```python
from build123d import *

# Parameters (mm, degrees)
SKETCH1_W                    = 40
SKETCH1_H                    = 60
SKETCH1_R                    = 2
BASE_FLANGE1_DEPTH           = 2
EDGE_FLANGE1_STRIP_W         = 9.4732
EDGE_FLANGE1_STRIP_H         = 2
EDGE_FLANGE1_STRIP_CUT_DEPTH = 40
EDGE_FLANGE1_DEPTH           = 40
SKETCH7_R                    = 2
CUT_EXTRUDE1_DEPTH           = 10


# Sheet-metal steps are written as plain solids
with BuildPart() as part:
    # Sketch1 → Base-Flange1 (new body)
    with BuildSketch(Plane.XY):
        with Locations((0, 30)):
            Rectangle(SKETCH1_W, SKETCH1_H)
        with Locations((-14, 50)):
            Circle(SKETCH1_R, mode=Mode.SUBTRACT)
        with Locations((0, 50)):
            Circle(SKETCH1_R, mode=Mode.SUBTRACT)
        with Locations((14, 50)):
            Circle(SKETCH1_R, mode=Mode.SUBTRACT)
        with Locations((-7, 40)):
            Circle(SKETCH1_R, mode=Mode.SUBTRACT)
        with Locations((7, 40)):
            Circle(SKETCH1_R, mode=Mode.SUBTRACT)
        with Locations((-14, 30)):
            Circle(SKETCH1_R, mode=Mode.SUBTRACT)
        with Locations((-7, 20)):
            Circle(SKETCH1_R, mode=Mode.SUBTRACT)
        with Locations((7, 20)):
            Circle(SKETCH1_R, mode=Mode.SUBTRACT)
        with Locations((0, 30)):
            Circle(SKETCH1_R, mode=Mode.SUBTRACT)
        with Locations((14, 30)):
            Circle(SKETCH1_R, mode=Mode.SUBTRACT)
        with Locations((-14, 10)):
            Circle(SKETCH1_R, mode=Mode.SUBTRACT)
        with Locations((0, 10)):
            Circle(SKETCH1_R, mode=Mode.SUBTRACT)
        with Locations((14, 10)):
            Circle(SKETCH1_R, mode=Mode.SUBTRACT)
    extrude(amount=-BASE_FLANGE1_DEPTH)

    # Edge-Flange1 strip (across the edge) → Edge-Flange1 strip cut (cut)
    with BuildSketch(Plane.YZ.offset(-20)):
        with Locations((-4, -1)):
            Rectangle(EDGE_FLANGE1_STRIP_W, EDGE_FLANGE1_STRIP_H)
    extrude(amount=EDGE_FLANGE1_STRIP_CUT_DEPTH, mode=Mode.SUBTRACT)

    # Edge-Flange1 section (across the edge) → Edge-Flange1 (add)
    with BuildSketch(Plane.YZ.offset(-20)):
        with BuildLine():
            Line((-2, 0.7366), (-2, 60))
            Line((-2, 60), (0, 60))
            Line((0, 60), (0, 0.7366))
            ThreePointArc((0, 0.7366), (0.215745145, 0.215745145), (0.7366, 0))
            Line((0.7366, 0), (0.7366, -2))
            ThreePointArc((0.7366, -2), (-1.198468417, -1.198468417), (-2, 0.7366))
        make_face()
    extrude(amount=EDGE_FLANGE1_DEPTH)

    # Sketch7 → Cut-Extrude1 (cut)
    with BuildSketch(Plane(origin=(0, 0, 0), x_dir=(1, 0, 0), z_dir=(0, 1, 0))):
        with Locations(Location((-14, -10.7366, 0), (0, 0, 270))):
            Circle(SKETCH7_R)
        with Locations(Location((0, -10.7366, 0), (0, 0, 270))):
            Circle(SKETCH7_R)
        with Locations(Location((14, -10.7366, 0), (0, 0, 270))):
            Circle(SKETCH7_R)
        with Locations(Location((-7, -20.7366, 0), (0, 0, 270))):
            Circle(SKETCH7_R)
        with Locations(Location((7, -20.7366, 0), (0, 0, 270))):
            Circle(SKETCH7_R)
        with Locations(Location((-14, -30.7366, 0), (0, 0, 270))):
            Circle(SKETCH7_R)
        with Locations(Location((0, -30.7366, 0), (0, 0, 270))):
            Circle(SKETCH7_R)
        with Locations(Location((14, -30.7366, 0), (0, 0, 270))):
            Circle(SKETCH7_R)
        with Locations(Location((-7, -40.7366, 0), (0, 0, 270))):
            Circle(SKETCH7_R)
        with Locations(Location((7, -40.7366, 0), (0, 0, 270))):
            Circle(SKETCH7_R)
        with Locations(Location((14, -50.7366, 0), (0, 0, 270))):
            Circle(SKETCH7_R)
        with Locations(Location((0, -50.7366, 0), (0, 0, 270))):
            Circle(SKETCH7_R)
        with Locations(Location((-14, -50.7366, 0), (0, 0, 270))):
            Circle(SKETCH7_R)
    extrude(amount=-CUT_EXTRUDE1_DEPTH, mode=Mode.SUBTRACT)


solid = part.part
```
Geometry check sheet. Reference: the model listing, model coordinates, mm. A direction names the side the tool comes from. Give positions to 0.01 mm unless a question says otherwise; leave off trailing zeros. Order: outer loops, then holes, each group sorted by start corner. A loop starts at its lowest first (then second) coordinate and runs counter-clockwise, first axis right, second up. Notation, with made-up numbers: (-16, 8) - (1, 8) arc R11 cw to (1, 26) - close; hole circle Ø7 at (-0.5, -15). An arc over 180 degrees is marked (long way). Write item = value, one per line. Start each with the question number.
1) Section check A-A (y = 40). Enter the section's corners in (x, z), then the cut area to 3 significant figures.
2) Gauge pin test, flat ends, axial feed: pin 1 Ø3 at (x, y) = (0, 10) entering from +Z; pin 2 Ø6.5 at (x, y) = (-7, 40) entering from +Z; pin 3 Ø20 at (x, z) = (-9.5, 41) entering from +Y. Record the tip position at first contact, or that the pin passes through.
3) Access from +Z, -Z, +X, -X, +Y, -Y to the whole of each face (thin tool, end or side, straight path). Record for faces 5 (the flat face through (4, 31, 0)), 6 (the cylindrical face through (14.601, -0.986, 52.644)).
4) Section check B-B (x = -14). Count the separate pieces of the cut face and the enclosed holes in it, then the cut area to 3 significant figures.
5) Section check C-C (y = 10). Enter the section's corners in (x, z), then the cut area to 3 significant figures.
6) Draft check along Z on faces 1 (the flat face through (0, -1, 60)), 2 (the cylindrical face through (0, 28, -1)), 3 (the flat face through (4, 31, -2)), 4 (the cylindrical face through (7.601, -0.986, 42.644)). Enter one of: released by +Z, released by -Z, zero draft, split by the parting line, or undercut.
7) Scan lines: L1, parallel to Y at x = 14, z = -0.65; L2, parallel to Y at x = -7.5, z = 9. Record each from-to range of solid material in increasing order.
8) Section check D-D (z = 10). Enter the section's corners in (x, y).
Geometry check:
q1.outline = (-20, -2) - (-9, -2) - (-9, 0) - (-20, 0) - close; (-5, -2) - (5, -2) - (5, 0) - (-5, 0) - close; (9, -2) - (20, -2) - (20, 0) - (9, 0) - close
q1.area = 64.0 mm2
q2.pin_1 = through
q2.pin_2 = 0
q2.pin_3 = 0
q3.face_5 = +Z, +X, -X, +Y
q3.face_6 = +Y, -Y
q4.separate_pieces = 7
q4.enclosed_holes = 0
q4.area = 195 mm2
q5.outline = (-20, -2) - (-16, -2) - (-16, 0) - (-20, 0) - close; (-12, -2) - (-2, -2) - (-2, 0) - (-12, 0) - close; (2, -2) - (12, -2) - (12, 0) - (2, 0) - close; (16, -2) - (20, -2) - (20, 0) - (16, 0) - close
q5.area = 56.0 mm2
q6.face_1 = released by +Z
q6.face_2 = zero draft
q6.face_3 = released by -Z
q6.face_4 = undercut
q7.L1 = -1.62 to 8, 12 to 28, 32 to 48, 52 to 60
q7.L2 = -2 to 0
q8.outline = (-20, -2) - (-15.86, -2) - (-15.86, 0) - (-20, 0) - close; (-12.14, -2) - (-1.86, -2) - (-1.86, 0) - (-12.14, 0) - close; (1.86, -2) - (12.14, -2) - (12.14, 0) - (1.86, 0) - close; (15.86, -2) - (20, -2) - (20, 0) - (15.86, 0) - close
